For this review, use the dimensioned drawing (mm, ordinates from the lowest corner) and the shaded views. A direction names the side the tool comes from. Coordinates: 2 decimals unless noted, no trailing zeros. Write each loop counter-clockwise with the first axis right and the second up, starting at its lowest first coordinate (ties: lowest second). Pieces come first, ordered by that corner, then holes. Notation, with made-up numbers: M 43.5,9.25 L 100.5,9.25 A23 ccw 100.5,31.25 Z; hole C 63.5,85.25 d5. An arc over 180 degrees is marked long. One line per question, with ' | ' between items.
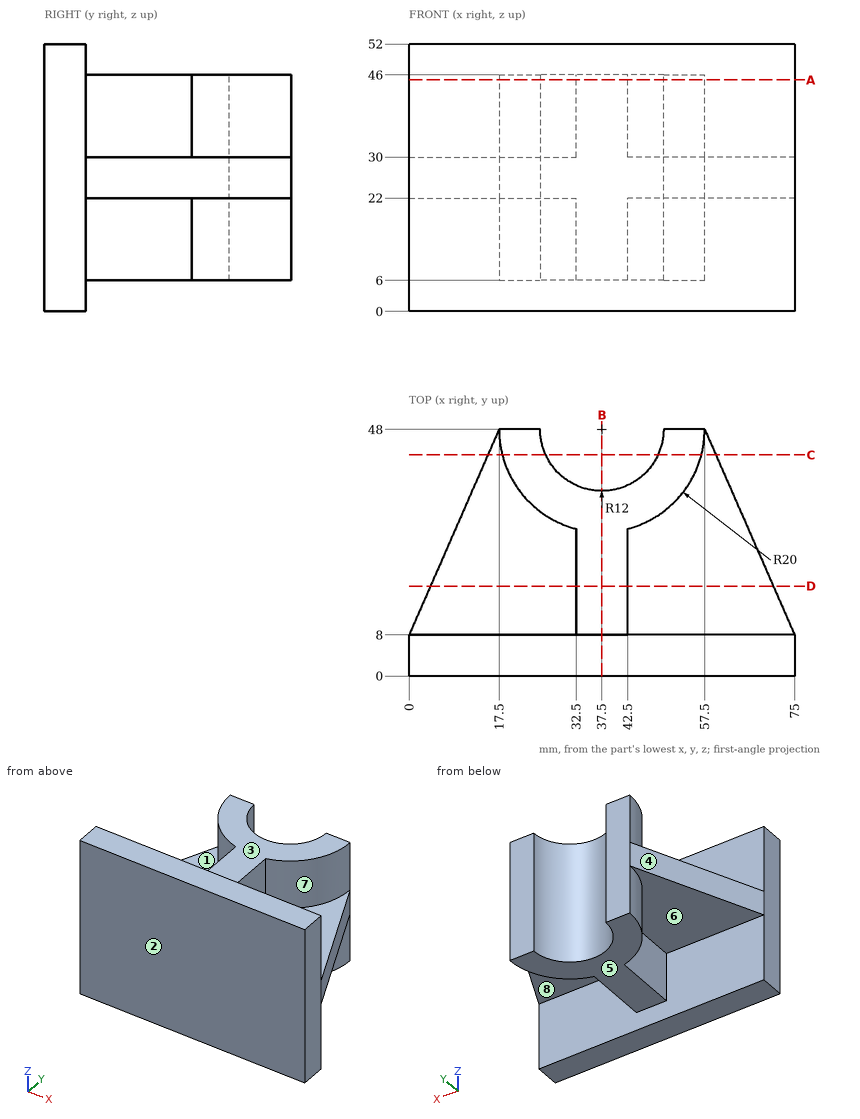
1) We need section C-C on y = 43. State the section outline as (x, z) points, then the cut area to 3 significant figures.
Responses:
outline: M 15.31,22 L 18.14,22 L 18.14,6 L 26.59,6 L 26.59,46 L 18.14,46 L 18.14,30 L 15.31,30 Z; M 48.41,6 L 56.86,6 L 56.86,22 L 59.69,22 L 59.69,30 L 56.86,30 L 56.86,46 L 48.41,46 Z | area: 722 mm^2
2) We need section A-A on z = 45. State the section outline as (x, y) points, then the cut area to 3 significant figures.
Responses:
outline: M 0,0 L 75,0 L 75,8 L 42.5,8 L 42.5,28.64 A20 ccw 57.5,48 L 49.5,48 A12 cw 25.5,48 L 17.5,48 A20 ccw 32.5,28.64 L 32.5,8 L 0,8 Z | area: 1,200 mm^2
3) We need section B-B on x = 37.5. State the section outline as (y, z) points.
Responses:
outline: M 0,0 L 8,0 L 8,6 L 36,6 L 36,46 L 8,46 L 8,52 L 0,52 Z
4) We need section D-D on y = 17.5. State the section outline as (x, z) points, then the cut area to 4 significant figures.
Responses:
outline: M 4.16,22 L 32.5,22 L 32.5,6 L 42.5,6 L 42.5,22 L 70.84,22 L 70.84,30 L 42.5,30 L 42.5,46 L 32.5,46 L 32.5,30 L 4.16,30 Z | area: 853.5 mm^2
5) The part is to be moulded in two halves that separate along Y. For the marked faces 1, 2, 3 and 4, say which applies: +Y half, -Y half, draft (parallel to the pull), parting line (faces both ways), or undercut.
Responses:
face 1: undercut | face 2: -Y half | face 3: draft | face 4: +Y half
6) Insertion check: pin 1 Ø20 at (x, y) = (28, 30.5) entering from -Z; pin 2 Ø3 at (x, y) = (58.5, 20.5) entering from -Z; pin 3 Ø13 at (y, z) = (19.5, 40.5) entering from -X. Each pin has a flat end and moves straight along its axis. Give the tip position at first contact, or say it passes through.
Responses:
pin 1: z = 6 | pin 2: z = 22 | pin 3: x = 32.5
7) To check wall thickness, follow line 1 along X through (y, z) = (28, 36.5); line 2 along X through (y, z) = (38, 27) (3 decimals); line 3 along Y through (x, z) = (29.5, 17.5). State the ranges of each line that lie inside material, in increasing order. Write a range as [from, to].
Responses:
line 1: [32.5, 42.5] | line 2: [13.125, 30.867], [44.133, 61.875] | line 3: [0, 8], [29.67, 39.06]
8) Machinability: for the marked faces 5, 6, 7 and 8, which of the approach directions +Z, -Z, +X, -X, +Y, -Y give a long, thin tool a straight path to every point of the face, cutting with its end or side? Answer none if there is none.
Responses:
face 5: -Z, +X, -X, +Y | face 6: -Z, -X | face 7: +Z, +X | face 8: -Z, +X
